Can you work these out from the model? Positions are in its coordinate system, mm. Face numbers are marked on the shaded views. A direction names the side the tool comes from. Give positions to 0.01 mm unless a question says otherwise; leave off trailing zeros. Write each loop counter-clockwise with the first axis right and the second up, starting at its lowest first coordinate (ties: lowest second). Pieces come first, ordered by that corner, then holes. Notation, with made-up numbers: M 58,7 L 73,7 A26 ccw 73,23 Z; hole C 50,68 d4. An arc over 180 degrees is marked long. Use CSV: the item, a comma, the result in double quotes. Start each with the question number.
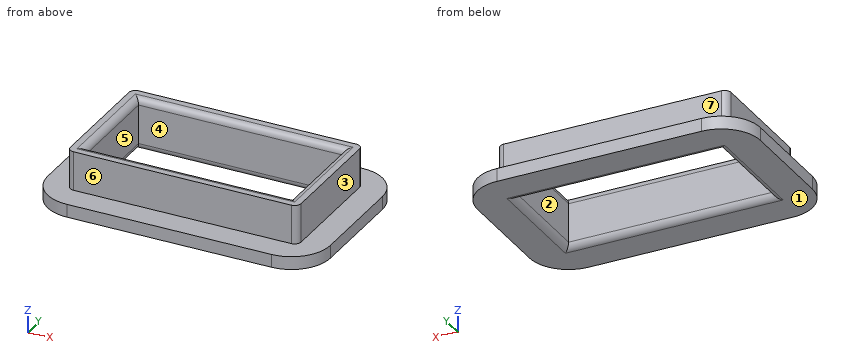
from build123d import *

# Parameters (mm, degrees)
F0_W     = 21.75
F0_H     = 13.8
F0_W_2   = 17.75
F0_H_2   = 9.8
F1_DEPTH = 1
F0_W_3   = 15.75
F0_H_3   = 7.8
F2_DEPTH = 4
F3_R     = 0.5
F4_R     = 0.5
F5_R     = 3


with BuildPart() as f1:
    # F0 (on Top) → F1 (new body)
    with BuildSketch(Plane.XY):
        with Locations((10.875, 6.9)):
            Rectangle(F0_W, F0_H)
        with Locations((10.875, 6.9)):
            Rectangle(F0_W_2, F0_H_2, mode=Mode.SUBTRACT)
    extrude(amount=F1_DEPTH)

    # F0 (on Top) → F2 (join)
    with BuildSketch(Plane.XY):
        with Locations((10.875, 6.9)):
            Rectangle(F0_W_2, F0_H_2)
        with Locations((10.875, 6.9)):
            Rectangle(F0_W_3, F0_H_3, mode=Mode.SUBTRACT)
    extrude(amount=F2_DEPTH)

    # F3
    f3_edges = [f1.edges().sort_by_distance(p)[0] for p in [
        (10.875, 10.8, 4),
        (18.75, 6.9, 4),
        (10.875, 3, 4),
        (3, 6.9, 4),
        (10.875, 10.8, 0),
        (3, 6.9, 0),
        (10.875, 3, 0),
        (18.75, 6.9, 0),
    ]]
    fillet(f3_edges, radius=F3_R)

    # F4
    f4_edges = [f1.edges().sort_by_distance(p)[0] for p in [
        (2, 11.8, 2.5),
        (2, 2, 2.5),
        (19.75, 2, 2.5),
        (19.75, 11.8, 2.5),
    ]]
    fillet(f4_edges, radius=F4_R)

    # F5
    f5_edges = [f1.edges().sort_by_distance(p)[0] for p in [
        (0, 13.8, 0.5),
        (21.75, 13.8, 0.5),
        (21.75, 0, 0.5),
        (0, 0, 0.5),
    ]]
    fillet(f5_edges, radius=F5_R)


solid = f1.part
(1) I want a section at A-A (x = 13.5). Write out the boundary of the cut face in (y, z).
(2) Which directions (+Z, -Z, +X, -X, +Y, -Y) give clear straight access to the entire face, cutting with the end or side of a thin tool? Please do the marked faces 5, 6 and 7.
(3) I want a section at D-D (x = 2.75). Write out the boundary of the cut face in (y, z), and give its area (3 significant figures).
(4) I want a section at B-B (y = 7). Write out the boundary of the cut face in (x, z).
(5) Please list where these lines run through material, in increasing order: L1, parallel to Y at x = 15.25, z = 1.3; L2, parallel to X at y = 10.5, z = 2.6; L3, parallel to Y at x = 8.5, z = 0.6. Write a range as [from, to].
(6) Thinking about a two-plate mould opening in X: for the marked faces 1, 2, 3 and 4, which applies, released by +X, released by -X, zero draft, split by the parting line, or undercut?
(7) Will these pins go through, and if not, where does the flat tip stop? pin 1 Ø7 at (x, y) = (7, 6) entering from +Z; pin 2 Ø0.9 at (x, z) = (13, 1.5) entering from +Y; pin 3 Ø1.5 at (x, z) = (17.5, 3) entering from -Y.
(8) I want a section at C-C (z = 3.2). Write out the boundary of the cut face in (x, y).
Geometry results:
1,outline,"M 0,0 L 2.5,0 A0.5 ccw 3,0.5 L 3,3.5 A0.5 ccw 2.5,4 L 2,4 L 2,1 L 0,1 Z; M 10.8,0.5 A0.5 ccw 11.3,0 L 13.8,0 L 13.8,1 L 11.8,1 L 11.8,4 L 11.3,4 A0.5 ccw 10.8,3.5 Z"
2,face 5,"+Z, -Z"
2,face 6,"+Z, +X, -X, -Y"
2,face 7,"+Z, +X, -X, +Y"
3,outline,"M 0.01,0 L 2.5,0 A0.5 ccw 2.75,0.07 L 11.05,0.07 A0.5 ccw 11.3,0 L 13.79,0 L 13.79,1 L 11.8,1 L 11.8,4 L 11.3,4 A0.5 ccw 11.05,3.93 L 2.75,3.93 A0.5 ccw 2.5,4 L 2,4 L 2,1 L 0.01,1 Z"
3,area,"42.0 mm2"
4,outline,"M 0,0 L 2.5,0 A0.5 ccw 3,0.5 L 3,3.5 A0.5 ccw 2.5,4 L 2,4 L 2,1 L 0,1 Z; M 18.75,0.5 A0.5 ccw 19.25,0 L 21.75,0 L 21.75,1 L 19.75,1 L 19.75,4 L 19.25,4 A0.5 ccw 18.75,3.5 Z"
5,L1,"y = [2, 3], [10.8, 11.8]"
5,L2,"x = [2, 3], [18.75, 19.75]"
5,L3,"y = [0, 3], [10.8, 13.8]"
6,face 1,"zero draft"
6,face 2,"undercut"
6,face 3,"released by +X"
6,face 4,"undercut"
7,pin 1,"stops at z = 4"
7,pin 2,"stops at y = 11.8"
7,pin 3,"stops at y = 2"
8,outline,"M 2,2.5 A0.5 ccw 2.5,2 L 19.25,2 A0.5 ccw 19.75,2.5 L 19.75,11.3 A0.5 ccw 19.25,11.8 L 2.5,11.8 A0.5 ccw 2,11.3 Z; hole M 3,3 L 18.75,3 L 18.75,10.8 L 3,10.8 Z"
